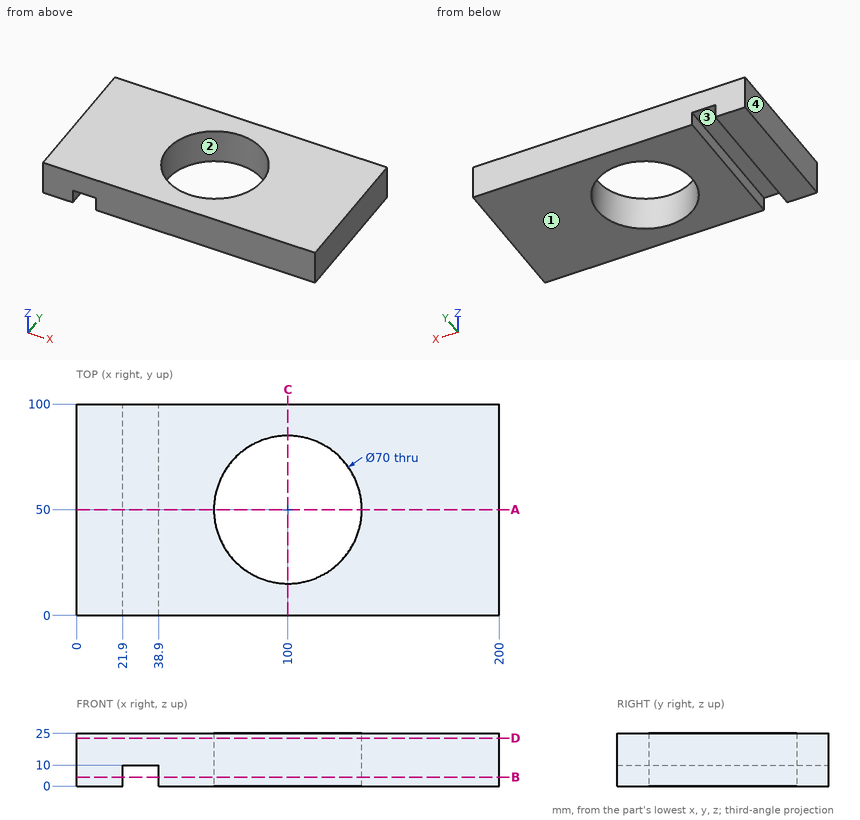
Design review of the part shown in the three views and the two pictorial views. Dimensions are in mm from the part's minimum x, y and z. Round coordinates to 2 decimals unless told otherwise and drop trailing zeros. Write each loop counter-clockwise with the first axis right and the second up, starting at its lowest first coordinate (ties: lowest second). Pieces come first, ordered by that corner, then holes. Notation, with made-up numbers: M -31,6 L -2,6 A28 ccw -2,44 Z; hole C 15,-2.5 d2. An arc over 180 degrees is marked long. One line per item, written item: value. Start each with the question number.
1. To check wall thickness, follow probe 1 along Y at (x, z) = (100, 5.75); probe 2 along X at (y, z) = (44, 19); probe 3 along Y at (x, z) = (78, 7). State the ranges of each line that lie inside material, in increasing order. Write a range as from..to.
2. Draft analysis for pull direction X (two halves, no side actions). For the marked faces 1, 2, 3 and 4, state which applies: pulls with the +X half, pulls with the -X half, needs draft (parallel to the pull), parting line crosses it, or undercut.
3. Clearance check with a flat-ended pin moving along its axis: P1, Ø5, axis at y = 41, z = 4, coming from the -X side. State where the tip first meets the part, or that it passes through.
4. Take a section at C-C on x = 100. State the section outline as (y, z) points.
5. Take a section at D-D on z = 22.75. State the section outline as (x, y) points, then the cut area to 3 significant figures.
6. Take a section at B-B on z = 4.25. State the section outline as (x, y) points, then the cut area to 3 significant figures.
7. Take a section at A-A on y = 50. State the section outline as (x, z) points, then the cut area to 3 significant figures.
Computed:
1. probe 1: y = 0..15, 85..100
1. probe 2: x = 0..65.52, 134.48..200
1. probe 3: y = 0..22.78, 77.22..100
2. face 1: needs draft
2. face 2: undercut
2. face 3: undercut
2. face 4: pulls with the -X half
3. P1: stops at x = 0
4. outline: M 0,0 L 15,0 L 15,25 L 0,25 Z; M 85,0 L 100,0 L 100,25 L 85,25 Z
5. outline: M 0,0 L 200,0 L 200,100 L 0,100 Z; hole C 100,50 d70
5. area: 16,200 mm²
6. outline: M 0,0 L 21.9,0 L 21.9,100 L 0,100 Z; M 38.9,0 L 200,0 L 200,100 L 38.9,100 Z; hole C 100,50 d70
6. area: 14,500 mm²
7. outline: M 0,0 L 21.9,0 L 21.9,10 L 38.9,10 L 38.9,0 L 65,0 L 65,25 L 0,25 Z; M 135,0 L 200,0 L 200,25 L 135,25 Z
7. area: 3,080 mm²
